Geometry: final body of the model. Coordinates: model frame, mm. Face numbers are marked on the shaded views. A direction names the side the tool comes from. Round coordinates to 2 decimals unless told otherwise and drop trailing zeros. Loops run counter-clockwise (first coordinate to the right, second up) from the corner with the lowest first, then second, coordinate; pieces in that order, holes last. Notation, with made-up numbers: (59, 35) - (76, 35) arc R28 ccw to (76, 74) - close; hole circle Ø9 at (35, 70). An arc over 180 degrees is marked (long way). Answer as a JSON object with one key per item and string values. Group by question number.
Item 1: Line query: line 1 (Y direction, x = -44, z = 6.5); line 2 (X direction, y = -3.5, z = 0.75); line 3 (X direction, y = -2.25, z = 2.25). Output: solid intervals per line, ascending.
Item 2: Section A-A (y = 5.25). Return the cut outline in (x, z).
Item 3: Reachability of the marked faces 1 and 2 from +Z, -Z, +X, -X, +Y, -Y: full face, straight path, thin tool, end or side. Return the list, or none.
Item 4: Section C-C (x = -39.5). Return the cut outline in (y, z), plus the area to 3 significant figures.
Item 5: Section B-B (x = -28). Return the cut outline in (y, z).
Item 6: First-contact query: pin 1 (0.8 mm diameter, centred on y = -4, z = 5.5, fed in from -X); pin 2 (4.5 mm diameter, centred on y = 4, z = 5, fed in from +X); pin 3 (1.5 mm diameter, centred on x = -38, y = -3.5, fed in from -Z); pin 4 (4 mm diameter, centred on x = -32.5, z = 4.5, fed in from +Y). Flat tips, straight axial feed; report the tip coordinate or a pass-through.
Item 7: Section D-D (y = 2). Return the cut outline in (x, z), plus the area to 3 significant figures.
Item 8: Draft query along X for the marked faces 3, 4, 5 and 6. Return one class per face: released by +X, released by -X, zero draft, split by the parting line, or undercut.
```python
from build123d import *

# Parameters (mm, degrees)
F0_R        = 2.4
F0_W        = 7.4481110471
F0_H        = 7.95
F1_DEPTH    = 7.88
F2_T1_DEPTH = 26.405


# Not quite as in the source:
# - a fillet or chamfer that OpenCascade refuses, or shapes differently, is made with other operations: its cross-section is extruded or revolved along the edge and cut away or added


with BuildPart() as f1:
    # F0 (on Top) → F1 (new body)
    with BuildSketch(Plane.XY):
        Polygon((-17.0395083171, 1.6058013724), (-28.7195083171, 1.6058013724), (-40.95139727, 1.6058013724), (-48.3995083171, 1.6058013724), (-48.3995083171, -5.7841986276), (-31.3221290569, -5.7841986276), (-17.0395083171, -5.7841986276), align=None)
        with Locations((-44.7195083171, -2.0891986276)):
            Circle(F0_R, mode=Mode.SUBTRACT)
        with Locations((-36.7195083171, -2.0891986276)):
            Circle(F0_R, mode=Mode.SUBTRACT)
        with BuildLine():
            ThreePointArc((-28.7195083171, -4.4891986276), (-31.1195083171, -2.0891986276), (-28.7195083171, 0.3108013724))
            ThreePointArc((-28.7195083171, 0.3108013724), (-26.3195083171, -2.0891986276), (-28.7195083171, -4.4891986276))
        make_face(mode=Mode.SUBTRACT)
        with BuildLine():
            ThreePointArc((-22.1195083171, -1.1891986276), (-21.7659549265, -1.0427520182), (-21.6195083171, -0.6891986276))
            Line((-21.6195083171, -0.6891986276), (-21.6195083171, 0.0671872376))
            ThreePointArc((-21.6195083171, 0.0671872376), (-21.601600524, 0.1242912617), (-21.5542909257, 0.1609431448))
            ThreePointArc((-21.5542909257, 0.1609431448), (-20.7195083171, 0.3108013724), (-19.8847257084, 0.1609431448))
            ThreePointArc((-19.8847257084, 0.1609431448), (-19.8374161101, 0.1242912617), (-19.8195083171, 0.0671872376))
            Line((-19.8195083171, 0.0671872376), (-19.8195083171, -0.6891986276))
            ThreePointArc((-19.8195083171, -0.6891986276), (-19.6730617076, -1.0427520182), (-19.3195083171, -1.1891986276))
            Line((-19.3195083171, -1.1891986276), (-18.5631224518, -1.1891986276))
            ThreePointArc((-18.5631224518, -1.1891986276), (-18.5060184277, -1.2071064207), (-18.4693665446, -1.2544160189))
            ThreePointArc((-18.4693665446, -1.2544160189), (-18.3572699449, -1.6651351029), (-18.3195083171, -2.0891986276))
            ThreePointArc((-18.3195083171, -2.0891986276), (-18.3572699449, -2.5132621524), (-18.4693665446, -2.9239812363))
            ThreePointArc((-18.4693665446, -2.9239812363), (-18.5060184277, -2.9712908345), (-18.5631224518, -2.9891986276))
            Line((-18.5631224518, -2.9891986276), (-19.3195083171, -2.9891986276))
            ThreePointArc((-19.3195083171, -2.9891986276), (-19.6730617076, -3.135645237), (-19.8195083171, -3.4891986276))
            Line((-19.8195083171, -3.4891986276), (-19.8195083171, -4.2455844929))
            ThreePointArc((-19.8195083171, -4.2455844929), (-19.8374161101, -4.302688517), (-19.8847257084, -4.3393404001))
            ThreePointArc((-19.8847257084, -4.3393404001), (-20.7195083171, -4.4891986276), (-21.5542909257, -4.3393404001))
            ThreePointArc((-21.5542909257, -4.3393404001), (-21.601600524, -4.302688517), (-21.6195083171, -4.2455844929))
            Line((-21.6195083171, -4.2455844929), (-21.6195083171, -3.4891986276))
            ThreePointArc((-21.6195083171, -3.4891986276), (-21.7659549265, -3.135645237), (-22.1195083171, -2.9891986276))
            Line((-22.1195083171, -2.9891986276), (-22.8758941823, -2.9891986276))
            ThreePointArc((-22.8758941823, -2.9891986276), (-22.9329982064, -2.9712908345), (-22.9696500895, -2.9239812363))
            ThreePointArc((-22.9696500895, -2.9239812363), (-23.0817466892, -2.5132621524), (-23.1195083171, -2.0891986276))
            ThreePointArc((-23.1195083171, -2.0891986276), (-23.0817466892, -1.6651351029), (-22.9696500895, -1.2544160189))
            ThreePointArc((-22.9696500895, -1.2544160189), (-22.9329982064, -1.2071064207), (-22.8758941823, -1.1891986276))
            Line((-22.8758941823, -1.1891986276), (-22.1195083171, -1.1891986276))
        make_face(mode=Mode.SUBTRACT)
        with Locations((-44.6754527935, 5.5808013724)):
            Rectangle(F0_W, F0_H)
        with Locations((-44.7195083171, 5.9108013724)):
            Circle(F0_R, mode=Mode.SUBTRACT)
    extrude(amount=F1_DEPTH)

    # F2: fillet of radius 3.705 on 5 edges, made by hand

    # F2_s2 → F2_t1 (cut)
    with BuildSketch(Plane.XY.offset(-9.2625)):
        with BuildLine():
            ThreePointArc((-44.6945083171, 9.5558013724), (-47.3143389413, 8.4706319967), (-48.3995083171, 5.8508013724))
            Line((-48.3995083171, 5.8508013724), (-48.3995083171, 9.5558013724))
            Line((-48.3995083171, 9.5558013724), (-44.6945083171, 9.5558013724))
        make_face()
        with BuildLine():
            ThreePointArc((-40.95139727, 5.8508013724), (-42.0365666457, 8.4706319967), (-44.65639727, 9.5558013724))
            Line((-44.65639727, 9.5558013724), (-40.95139727, 9.5558013724))
            Line((-40.95139727, 9.5558013724), (-40.95139727, 5.8508013724))
        make_face()
        with BuildLine():
            ThreePointArc((-48.3995083171, -2.0791986276), (-47.3143389413, -4.6990292519), (-44.6945083171, -5.7841986276))
            Line((-44.6945083171, -5.7841986276), (-48.3995083171, -5.7841986276))
            Line((-48.3995083171, -5.7841986276), (-48.3995083171, -2.0791986276))
        make_face()
        with BuildLine():
            ThreePointArc((-17.0395083171, -2.0991986276), (-18.1246776928, 0.5206319967), (-20.7445083171, 1.6058013724))
            Line((-20.7445083171, 1.6058013724), (-17.0395083171, 1.6058013724))
            Line((-17.0395083171, 1.6058013724), (-17.0395083171, -2.0991986276))
        make_face()
        with BuildLine():
            ThreePointArc((-17.0395083171, -2.0791986276), (-18.1246776928, -4.6990292519), (-20.7445083171, -5.7841986276))
            Line((-20.7445083171, -5.7841986276), (-17.0395083171, -5.7841986276))
            Line((-17.0395083171, -5.7841986276), (-17.0395083171, -2.0791986276))
        make_face()
    extrude(amount=F2_T1_DEPTH, mode=Mode.SUBTRACT)


solid = f1.part
```
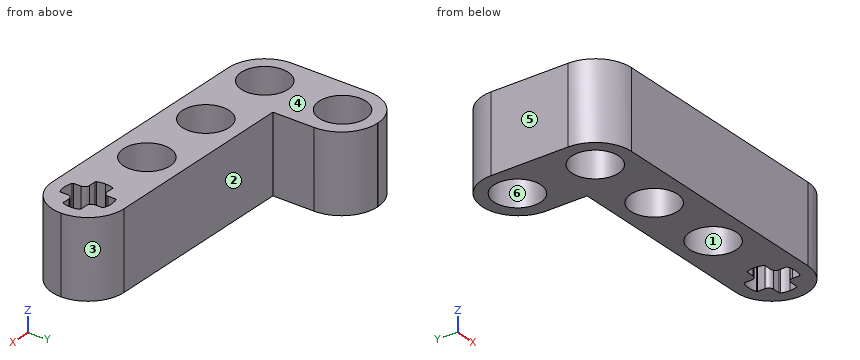
Values:
{
 "1": {"line 1": "y = -5.78 to -4.38, 0.2 to 3.62, 8.2 to 9.5", "line 2": "x = -48.12 to -46.66, -42.78 to -38.66, -34.78 to -30.66, -26.78 to -21.62, -19.82 to -17.32", "line 3": "x = -48.4 to -47.11, -42.32 to -39.11, -34.32 to -31.11, -26.32 to -23.11, -18.32 to -17.04"},
 "2": {"outline": "(-48.4, 0) - (-47.03, 0) - (-47.03, 7.88) - (-48.4, 7.88) - close; (-42.41, 0) - (-40.95, 0) - (-40.95, 7.88) - (-42.41, 7.88) - close"},
 "3": {"face 1": "+Z, -Z", "face 2": "+Z, -Z, +X, +Y"},
 "4": {"outline": "(-5.78, 0) - (1.61, 0) - (1.61, 7.88) - (-5.78, 7.88) - close", "area": "58.2 mm^2"},
 "5": {"outline": "(-5.78, 0) - (-4.38, 0) - (-4.38, 7.88) - (-5.78, 7.88) - close; (0.2, 0) - (1.61, 0) - (1.61, 7.88) - (0.2, 7.88) - close"},
 "6": {"pin 1": "stops at x = -48.07", "pin 2": "stops at x = -40.95", "pin 3": "stops at z = 0", "pin 4": "stops at y = 1.61"},
 "7": {"outline": "(-48.4, 0) - (-40.95, 0) - (-40.95, 7.88) - (-48.4, 7.88) - close", "area": "58.7 mm^2"},
 "8": {"face 3": "released by +X", "face 4": "zero draft", "face 5": "released by -X", "face 6": "undercut"}
}
